from build123d import *

# Parameters (mm, degrees)
WYCI_GNI_CIE_CIENKA_CIANKA1_DEPTH      = 400
WYCI_GNI_CIE_CIENKA_CIANKA1_DEPTH_BACK = 400


with BuildPart() as part:
    # Szkic3 → Wyciągnięcie-cienka ścianka1 (new, two sides)
    with BuildSketch(Plane(origin=(0, 0, 0), x_dir=(1, 0, 0), z_dir=(0, 1, 0))) as wyci_gni_cie_cienka_cianka1_sk:
        Polygon((956.655966162, -465.583132528), (969.891434648, -477.079346089), (970.078511471, -618.499346089), (1360.07269303, -618.499346089), (1360.07269303, -618.999346089), (969.579172456, -618.999346089), (969.391736143, -477.307590729), (956.328086187, -465.960617259), align=None)
    extrude(amount=WYCI_GNI_CIE_CIENKA_CIANKA1_DEPTH)
    extrude(wyci_gni_cie_cienka_cianka1_sk.sketch, amount=-WYCI_GNI_CIE_CIENKA_CIANKA1_DEPTH_BACK)

    # Cięcie powierzchnią1
    split(bisect_by=Plane(origin=(90.906039695, -464.075841363, 0), x_dir=(-0.9813493581662637, -0.19223276834780917, 0), z_dir=(-0.19223276834780917, 0.9813493581662637, 0)), keep=Keep.TOP)

    # Cięcie powierzchnią2
    split(bisect_by=Plane(origin=(90.906039695, 464.075841363, 0), x_dir=(-0.9813493581662637, 0.19223276834780917, 0), z_dir=(0.19223276834780917, 0.9813493581662637, 0)), keep=Keep.BOTTOM)


solid = part.part
Source: CAD feature listing. Evaluate the final solid. Frame: model axes, mm. A direction names the side the tool comes from. Coordinates: 2 decimals unless noted, no trailing zeros. Loops run counter-clockwise (first coordinate to the right, second up) from the corner with the lowest first, then second, coordinate; pieces in that order, holes last. Notation, with made-up numbers: (-40, 46.25) - (5, 46.25) arc R22 cw to (5, 70.25) - close; hole circle Ø9 at (6, -20). An arc over 180 degrees is marked (long way). One line per question, with ' | ' between items.
1) First-contact query: P1, Ø4, axis at y = -173, z = 506.5, coming from the +X side; P2, Ø2, axis at x = 1194.5, y = 15, coming from the -Z side; P3, Ø8, axis at y = 146, z = 595.5, coming from the +X side. Flat tips, straight axial feed; report the tip coordinate or a pass-through.
Report:
P1: stops at x = 969.93 | P2: stops at z = 618.5 | P3: stops at x = 970.05
2) Section B-B, the plane z = 484.5. Return loops of the section in (x, y).
Report:
outline: (969.4, -291.99) - (969.9, -291.89) - (969.9, 291.89) - (969.4, 291.99) - close
3) Section A-A, the plane y = 138. Return loops of the section in (x, z), then the cut area to 3 significant figures.
Report:
outline: (956.33, 465.96) - (956.66, 465.58) - (969.89, 477.08) - (970.08, 618.5) - (1360.07, 618.5) - (1360.07, 619) - (969.58, 619) - (969.39, 477.31) - close | area: 275 mm²
4) Section C-C, the plane x = 1060.5. Return loops of the section in (y, z).
Report:
outline: (-274.15, 618.5) - (274.15, 618.5) - (274.15, 619) - (-274.15, 619) - close
5) Line query: line 1 along X through (y, z) = (-145, 492); line 2 along X through (y, z) = (269, 607.5); line 3 along Z through (x, y) = (1312, 105). Output: solid intervals per line, ascending.
Report:
line 1: x = 969.41 to 969.91 | line 2: x = 969.56 to 970.06 | line 3: z = 618.5 to 619
6) Set-up query: faces 1 (the face through (1168, 4, 618.999)), 2 (the face through (1162, 4, 618.499)). Return all of +Z, -Z, +X, -X, +Y, -Y with unobstructed straight access to the full face (end or side cutting, diameter ignored); none if empty.
Report:
face 1: +Z, +X, -X, +Y, -Y | face 2: -Z, +X, +Y, -Y
7) Section D-D, the plane y = 235. Return loops of the section in (x, z).
Report:
outline: (956.33, 465.96) - (956.66, 465.58) - (969.89, 477.08) - (970.08, 618.5) - (1260.34, 618.5) - (1260.34, 619) - (969.58, 619) - (969.39, 477.31) - close
